CAD build for the part. Positions are in the model's coordinates, mm. Face numbers are marked on the shaded views. A direction names the side the tool comes from. Give positions to 0.01 mm unless a question says otherwise; leave off trailing zeros. Write each loop counter-clockwise with the first axis right and the second up, starting at its lowest first coordinate (ties: lowest second). Pieces come first, ordered by that corner, then holes. Notation, with made-up numbers: (-6.5, 59) - (31.5, 59) arc R15 ccw to (31.5, 87) - close; hole circle Ø7 at (11, -32). An arc over 180 degrees is marked (long way). Write item = value, one per line. Start each with the question number.
```python
from build123d import *

# Parameters (mm, degrees)
SKETCH1_R           = 10.16
SKETCH1_R_2         = 1.625
BOSS_EXTRUDE2_DEPTH = 1.778
SKETCH3_R           = 3.625
SKETCH3_R_2         = 2.5
BOSS_EXTRUDE3_DEPTH = 4.572
SKETCH4_R           = 1.25
CUT_EXTRUDE1_DEPTH  = 7.35


with BuildPart() as part:
    # Sketch1 → Boss-Extrude2 (new body)
    with BuildSketch(Plane(origin=(0, 0, 0), x_dir=(1, 0, 0), z_dir=(0, 1, 0))):
        Circle(SKETCH1_R)
        Circle(SKETCH1_R_2, mode=Mode.SUBTRACT)
    extrude(amount=BOSS_EXTRUDE2_DEPTH)

    # Sketch3 → Boss-Extrude3 (add)
    with BuildSketch(Plane(origin=(0, 1.778, 0), x_dir=(1, 0, 0), z_dir=(0, 1, 0))):
        Circle(SKETCH3_R)
        Circle(SKETCH3_R_2, mode=Mode.SUBTRACT)
    extrude(amount=BOSS_EXTRUDE3_DEPTH)

    # Sketch4 → Cut-Extrude1 (cut, through all)
    with BuildSketch(Plane.XZ):
        with Locations((0, 7.31)):
            Circle(SKETCH4_R)
        with Locations((7.31, 0)):
            Circle(SKETCH4_R)
        with Locations((-7.31, 0)):
            Circle(SKETCH4_R)
        with Locations((0, -7.31)):
            Circle(SKETCH4_R)
    extrude(amount=-CUT_EXTRUDE1_DEPTH, mode=Mode.SUBTRACT)


solid = part.part
```
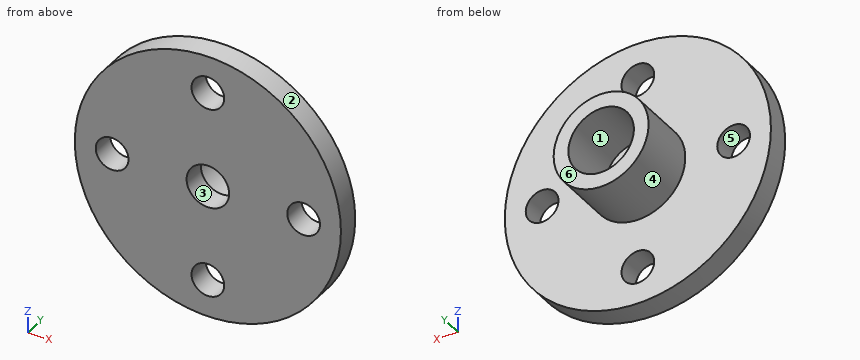
1. Tool access for the marked faces 1 and 2: list every direction of +Z, -Z, +X, -X, +Y, -Y with a clear straight run to the whole face (end or side of a thin tool).
2. Cut at C-C (y = 1). Give the cut face in (x, z) (3 decimals).
3. Cut at A-A (z = 0). Give the cut face in (x, y) (3 decimals), then the cut area to 3 significant figures.
4. Pin check, flat tips, straight feed: pin 1 Ø2 at (x, z) = (0, -7.31) entering from -Y; pin 2 Ø4 at (x, z) = (-7.31, 0) entering from +Y. Stop position of each tip, or through.
5. Mould opens along Z. For the marked faces 3, 4, 5 and 6 say: +Z half, -Z half, draft (parallel to the pull), parting line (faces both ways), or undercut.
6. Cut at B-B (x = 0). Give the cut face in (y, z) (3 decimals), then the cut area to 3 significant figures.
7. Wall check: line 1 along Z through (x, y) = (0, 0.65) (3 decimals); line 2 along Z through (x, y) = (0, 3.8) (3 decimals); line 3 along Y through (x, z) = (-5, -3). Give the ranges that are in metal, low to high.
8. Cut at D-D (x = -8). Give the cut face in (y, z), then the cut area to 3 significant figures.
Output:
q1.face_1 = +Y
q1.face_2 = +Y, -Y
q2.outline = circle Ø20.32 at (0, 0); hole circle Ø2.5 at (-7.31, 0); hole circle Ø3.25 at (0, 0); hole circle Ø2.5 at (0, -7.31); hole circle Ø2.5 at (0, 7.31); hole circle Ø2.5 at (7.31, 0)
q3.outline = (-10.16, 0) - (-8.56, 0) - (-8.56, 1.778) - (-10.16, 1.778) - close; (-6.06, 0) - (-1.625, 0) - (-1.625, 1.778) - (-2.5, 1.778) - (-2.5, 6.35) - (-3.625, 6.35) - (-3.625, 1.778) - (-6.06, 1.778) - close; (1.625, 0) - (6.06, 0) - (6.06, 1.778) - (3.625, 1.778) - (3.625, 6.35) - (2.5, 6.35) - (2.5, 1.778) - (1.625, 1.778) - close; (8.56, 0) - (10.16, 0) - (10.16, 1.778) - (8.56, 1.778) - close
q3.area = 31.7 mm2
q4.pin_1 = through
q4.pin_2 = 1.78
q5.face_3 = undercut
q5.face_4 = parting line
q5.face_5 = undercut
q5.face_6 = draft
q6.outline = (0, -10.16) - (1.778, -10.16) - (1.778, -8.56) - (0, -8.56) - close; (0, -6.06) - (1.778, -6.06) - (1.778, -3.625) - (6.35, -3.625) - (6.35, -2.5) - (1.778, -2.5) - (1.778, -1.625) - (0, -1.625) - close; (0, 1.625) - (1.778, 1.625) - (1.778, 2.5) - (6.35, 2.5) - (6.35, 3.625) - (1.778, 3.625) - (1.778, 6.06) - (0, 6.06) - close; (0, 8.56) - (1.778, 8.56) - (1.778, 10.16) - (0, 10.16) - close
q6.area = 31.7 mm2
q7.line_1 = -10.16 to -8.56, -6.06 to -1.625, 1.625 to 6.06, 8.56 to 10.16
q7.line_2 = -3.625 to -2.5, 2.5 to 3.625
q7.line_3 = 0 to 1.78
q8.outline = (0, -6.26) - (1.78, -6.26) - (1.78, -1.04) - (0, -1.04) - close; (0, 1.04) - (1.78, 1.04) - (1.78, 6.26) - (0, 6.26) - close
q8.area = 18.6 mm2
